Source: CAD feature listing. Evaluate the final solid. Frame: model axes, mm. Face numbers are marked on the shaded views. A direction names the side the tool comes from. Give positions to 0.01 mm unless a question says otherwise; leave off trailing zeros. Write each loop counter-clockwise with the first axis right and the second up, starting at its lowest first coordinate (ties: lowest second). Pieces come first, ordered by that corner, then holes. Notation, with made-up numbers: (-11, 89) - (36, 89) arc R21 cw to (36, 126) - close; hole circle Ø1 at (54, 23). An arc over 180 degrees is marked (long way). Answer as a JSON object with one key per item and string values. Group by question number.
from build123d import *

# Parameters (mm, degrees)
SKETCH2_W           = 80
SKETCH2_H           = 100
BOSS_EXTRUDE1_DEPTH = 40
SKETCH3_W           = 40
SKETCH3_H           = 12.05
CUT_EXTRUDE1_DEPTH  = 8
SKETCH5_R           = 1.4
CUT_EXTRUDE2_DEPTH  = 2
SKETCH8_W           = 100
SKETCH8_H           = 40
CUT_EXTRUDE5_DEPTH  = 30
SKETCH9_W           = 50
SKETCH9_H           = 40
CUT_EXTRUDE6_DEPTH  = 40


with BuildPart() as part:
    # Sketch2 → Boss-Extrude1 (new body)
    with BuildSketch(Plane(origin=(0, 0, 0), x_dir=(1, 0, 0), z_dir=(0, 1, 0))):
        Rectangle(SKETCH2_W, SKETCH2_H)
    extrude(amount=BOSS_EXTRUDE1_DEPTH)

    # Sketch3 → Cut-Extrude1 (cut)
    with BuildSketch(Plane(origin=(0, 40, 0), x_dir=(1, 0, 0), z_dir=(0, 1, 0))):
        with Locations((20, 0)):
            Rectangle(SKETCH3_W, SKETCH3_H)
    extrude(amount=-CUT_EXTRUDE1_DEPTH, mode=Mode.SUBTRACT)

    # Sketch5 → Cut-Extrude2 (cut)
    with BuildSketch(Plane(origin=(0, 40, 0), x_dir=(1, 0, 0), z_dir=(0, 1, 0))):
        with Locations(Location((6, 21.725, 0), (0, 0, 270))):
            Circle(SKETCH5_R)
        with Locations(Location((32, 21.725, 0), (0, 0, 270))):
            Circle(SKETCH5_R)
        with Locations(Location((32, 34.725, 0), (0, 0, 270))):
            Circle(SKETCH5_R)
        with Locations(Location((6, 34.725, 0), (0, 0, 270))):
            Circle(SKETCH5_R)
    extrude(amount=-CUT_EXTRUDE2_DEPTH, mode=Mode.SUBTRACT)

    # Sketch8 → Cut-Extrude5 (cut)
    with BuildSketch(Plane.ZY.offset(40)):
        with Locations((0, 20)):
            Rectangle(SKETCH8_W, SKETCH8_H)
    extrude(amount=-CUT_EXTRUDE5_DEPTH, mode=Mode.SUBTRACT)

    # Sketch9 → Cut-Extrude6 (cut)
    with BuildSketch(Plane.XY.offset(50)):
        with Locations((15, 20)):
            Rectangle(SKETCH9_W, SKETCH9_H)
    extrude(amount=-CUT_EXTRUDE6_DEPTH, mode=Mode.SUBTRACT)


solid = part.part
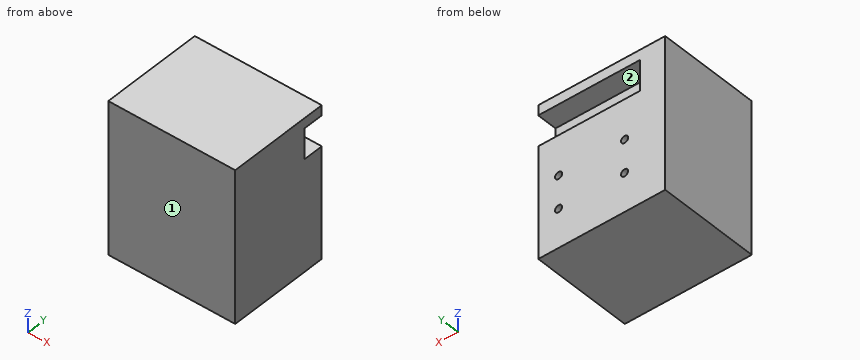
Q1. Section D-D on x = 32. Return the cut outline in (y, z) (3 decimals), then the cut area to 3 significant figures.
Q2. Section C-C on z = -0.5. Return the cut outline in (x, y), then the cut area to 3 significant figures.
Q3. Section B-B on y = 36. Return the cut outline in (x, z) (3 decimals).
Q4. Section A-A on x = 20.5. Return the cut outline in (y, z) (3 decimals).
Q5. Ray query, probe 1 along Y at (x, z) = (37, 2.5). Return the intervals inside material, ascending. Write a range as [from, to].
Q6. Reachability of the marked faces 1 and 2 from +Z, -Z, +X, -X, +Y, -Y: full face, straight path, thin tool, end or side. Return the list, or none.
Q7. First-contact query: pin 1 Ø0.8 at (x, z) = (32.5, -35) entering from +Y; pin 2 Ø6.5 at (y, z) = (36, 0.5) entering from +X; pin 3 Ø3.5 at (x, z) = (20, -2.5) entering from +Y. Flat tips, straight axial feed; report the tip coordinate or a pass-through.
Taken from the geometry:
{
 "1": {"outline": "(0, -50) - (40, -50) - (40, -36.125) - (38, -36.125) - (38, -33.325) - (40, -33.325) - (40, -23.125) - (38, -23.125) - (38, -20.325) - (40, -20.325) - (40, -6.025) - (32, -6.025) - (32, 6.025) - (40, 6.025) - (40, 10) - (0, 10) - close", "area": "2,290 mm²"},
 "2": {"outline": "(-10, 0) - (40, 0) - (40, 32) - (0, 32) - (0, 40) - (-10, 40) - close", "area": "1,680 mm²"},
 "3": {"outline": "(-10, -50) - (40, -50) - (40, -6.025) - (0, -6.025) - (0, 6.025) - (40, 6.025) - (40, 10) - (-10, 10) - close"},
 "4": {"outline": "(0, -50) - (40, -50) - (40, -6.025) - (32, -6.025) - (32, 6.025) - (40, 6.025) - (40, 10) - (0, 10) - close"},
 "5": {"probe 1": "y = [0, 32]"},
 "6": {"face 1": "+Z, -Z, +X, -X, -Y", "face 2": "+X, +Y"},
 "7": {"pin 1": "stops at y = 38", "pin 2": "stops at x = 0", "pin 3": "stops at y = 32"}
}
